Geometry check sheet. Reference: the model listing, model coordinates, mm. Face numbers are marked on the shaded views. Give positions to 0.01 mm unless a question says otherwise; leave off trailing zeros. Write each loop counter-clockwise with the first axis right and the second up, starting at its lowest first coordinate (ties: lowest second). Pieces come first, ordered by that corner, then holes. Notation, with made-up numbers: M 1,23.25 L 10,23.25 A5 ccw 10,32.25 Z; hole C 54,-36 d5. An arc over 180 degrees is marked long. Use one line per item in the form item = value. Start each with the question number.
```python
from build123d import *

# Parameters (mm, degrees)
F0_R     = 100
F1_DEPTH = 28
F2_T     = -2
F3_R     = 1
F4_DEPTH = 21
F5_R     = 1
F6_DEPTH = 14


with BuildPart() as f1:
    # F0 (on Top) → F1 (new body)
    with BuildSketch(Plane.XY):
        Circle(F0_R)
    extrude(amount=F1_DEPTH)

    # F2
    f2_openings = [f1.faces().sort_by_distance(p)[0] for p in [
        (0, 0, 28),
    ]]
    offset(amount=F2_T, openings=f2_openings)

    # F3 (on face) → F4 (join)
    with BuildSketch(Plane.XY.offset(2)):
        Circle(F3_R)
    extrude(amount=F4_DEPTH)

    # F5 (on face) → F6 (join)
    with BuildSketch(Plane.XY.offset(2)):
        with Locations((48, 0)):
            Circle(F5_R)
    extrude(amount=F6_DEPTH)


solid = f1.part
```
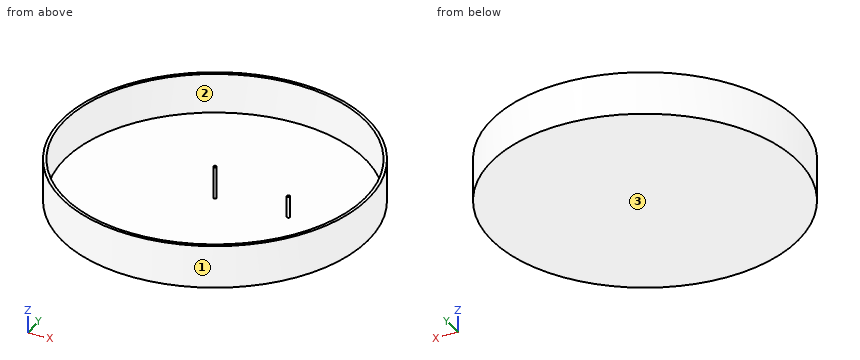
(1) Depth check by flat-ended pin: pin 1 (2 mm diameter, centred on y = 17, z = 22.5, fed in from +X); pin 2 (1.6 mm diameter, centred on x = 47.5, y = 0, fed in from +Z); pin 3 (2 mm diameter, centred on x = 5.5, y = 1.5, fed in from +Z). Enter the tip coordinate at first touch or a pass-through.
(2) Draft check along Y on the marked faces 1, 2 and 3. Enter one of: released by +Y, released by -Y, zero draft, split by the parting line, or undercut.
(3) Sectioned sample at C-C, the plane y = 83.5. Record the boundary of the cut face in (x, z) (3 decimals), plus the area to 3 significant figures.
(4) Thickness scan on probe 1 along Y at (x, z) = (0, 9.5); probe 2 along Z at (x, y) = (21.5, -80.5); probe 3 along X at (y, z) = (90.5, 6.75). Record the ranges inside material, lowest first. Write a range as [from, to].
(5) Sectioned sample at B-B, the plane x = 30.5. Record the boundary of the cut face in (y, z).
(6) Sectioned sample at A-A, the plane z = 10.5. Record the boundary of the cut face in (x, y).
Numbers:
q1.pin_1 = 98.71
q1.pin_2 = 16
q1.pin_3 = 2
q2.face_1 = split by the parting line
q2.face_2 = undercut
q2.face_3 = zero draft
q3.outline = M -55.025,0 L 55.025,0 L 55.025,28 L 51.301,28 L 51.301,2 L -51.301,2 L -51.301,28 L -55.025,28 Z
q3.area = 414 mm2
q4.probe_1 = [-100, -98], [-1, 1], [98, 100]
q4.probe_2 = [0, 2]
q4.probe_3 = [-42.54, -37.6], [37.6, 42.54]
q5.outline = M -95.24,0 L 95.24,0 L 95.24,28 L 93.13,28 L 93.13,2 L -93.13,2 L -93.13,28 L -95.24,28 Z
q6.outline = C 0,0 d200; C 0,0 d2; C 48,0 d2; hole C 0,0 d196
